Geometry check sheet. Reference: the model listing, model coordinates, mm. A direction names the side the tool comes from. Coordinates: 2 decimals unless noted, no trailing zeros. Order: outer loops, then holes, each group sorted by start corner. A loop starts at its lowest first (then second) coordinate and runs counter-clockwise, first axis right, second up. Notation, with made-up numbers: (-0.75, 32.5) - (52.25, 32.5) arc R14 cw to (52.25, 59.5) - close; hole circle Ø2 at (-35, 73.5). An arc over 180 degrees is marked (long way). Return JSON: item names as keys, results as strings. Group by question number.
Item 1: Section check C-C on x = -11. Enter the section's corners in (y, z), then the cut area to 3 significant figures.
Item 2: Gauge pin test, flat ends, axial feed: pin 1 (3.5 mm diameter, centred on x = -4.95, y = -4.95, fed in from +Z); pin 2 (1 mm diameter, centred on y = 0, z = 13, fed in from +X); pin 3 (4 mm diameter, centred on y = 10, z = 15.5, fed in from -X); pin 4 (2.5 mm diameter, centred on x = -8, z = 15, fed in from -Y). Record the tip position at first contact, or that the pin passes through.
Item 3: Scan lines: probe 1 along Y at (x, z) = (-1.4, 16); probe 2 along Y at (x, z) = (-5, 2.25); probe 3 along Y at (x, z) = (-0.75, 13.75). Record each from-to range of solid material in increasing order.
Item 4: Section check D-D on x = -2. Enter the section's corners in (y, z).
Item 5: Section check B-B on z = 16. Enter the section's corners in (x, y), then the cut area to 4 significant figures.
Item 6: Tool access check on faces 1 (the cylindrical face through (-10, 0, 7)), 2 (the flat face through (-4, 9.96, 14.98)), 3 (the flat face through (-5, 0, 14)). Record the directions out of +Z, -Z, +X, -X, +Y, -Y that give a thin tool (end or side, any length) a straight path to the whole face; none if there is none.
Item 7: Section check A-A on y = 10.5. Enter the section's corners in (x, z), then the cut area to 4 significant figures.
Item 8: Draft check along Y on faces 4 (the flat face through (-8, -7.5, 16)), 5 (the flat face through (-5, 0, 3)), 6 (the flat face through (0, 10.2, 8.9)). Enter one of: pulls with the +Y half, pulls with the -Y half, needs draft (parallel to the pull), parting line crosses it, or undercut.
from build123d import *

# Parameters (mm, degrees)
SKETCH_1_W               = 25
SKETCH_1_H               = 25
EXTRUDE_1_DEPTH          = 10
SKETCH_2_R               = 10
CUT_EXTRUDE_1_DEPTH      = 7
SKETCH_3_R               = 4.5
CUT_EXTRUDE_2_DEPTH      = 20.013153342
SKETCH_4_R               = 2
CUT_EXTRUDE_4_DEPTH      = 20.013153342
PATTERN_CIRCULAR_1_COUNT = 4
SKETCH_5_W               = 25
SKETCH_5_H               = 25
EXTRUDE_2_DEPTH          = 8
SKETCH_6_W               = 10
SKETCH_6_H               = 10
CUT_EXTRUDE_5_DEPTH      = 8
SKETCH_8_W               = 17.447834749
SKETCH_8_H               = 20.945056097
CUT_EXTRUDE_8_DEPTH      = 34.24530042
CUT_EXTRUDE_START        = -4
SKETCH_12_W              = 5
SKETCH_12_H              = 5
CUT_EXTRUDE_9_DEPTH      = 22.228951623
SKETCH_13_R              = 1
CUT_EXTRUDE_10_DEPTH     = 24.505318547


with BuildPart() as part:
    # 草图1 → 凸台-拉伸1 (new body)
    with BuildSketch(Plane.XY):
        Rectangle(SKETCH_1_W, SKETCH_1_H)
    extrude(amount=EXTRUDE_1_DEPTH)

    # 草图2 → 切除-拉伸1 (cut)
    with BuildSketch(Plane.XY.offset(10)):
        Circle(SKETCH_2_R)
    extrude(amount=-CUT_EXTRUDE_1_DEPTH, mode=Mode.SUBTRACT)

    # 草图3 → 切除-拉伸2 (cut, through all)
    with BuildSketch(Plane.XY.offset(3)):
        Circle(SKETCH_3_R)
    extrude(amount=-CUT_EXTRUDE_2_DEPTH, mode=Mode.SUBTRACT)

    # 草图4 → 切除-拉伸4 (cut, through all)
    with BuildSketch(Plane.XY.offset(3)):
        with Locations((-4.949747468, 4.949747468)):
            Circle(SKETCH_4_R)
    cut_extrude_4 = extrude(amount=-CUT_EXTRUDE_4_DEPTH, mode=Mode.SUBTRACT)

    # 阵列(圆周)1: 切除-拉伸4 ×4 about axis
    pattern_circular_1_axis = Axis((0, 0, 0), (0, 0, 1))
    for i in range(1, PATTERN_CIRCULAR_1_COUNT):
        add(cut_extrude_4.rotate(pattern_circular_1_axis, i * 360 / PATTERN_CIRCULAR_1_COUNT), mode=Mode.SUBTRACT)

    # 草图5 → 凸台-拉伸2 (add)
    with BuildSketch(Plane.XY.offset(10)):
        Rectangle(SKETCH_5_W, SKETCH_5_H)
    extrude(amount=EXTRUDE_2_DEPTH)

    # 草图6 → 切除-拉伸5 (cut)
    with BuildSketch(Plane.XY.offset(18)):
        Rectangle(SKETCH_6_W, SKETCH_6_H)
    extrude(amount=-CUT_EXTRUDE_5_DEPTH, mode=Mode.SUBTRACT)

    # 草图8 → 切除-拉伸8 (cut, through all)
    with BuildSketch(Plane.XZ.offset(12.5)):
        with Locations((8.723917375, 10.472528049)):
            Rectangle(SKETCH_8_W, SKETCH_8_H)
    extrude(amount=-CUT_EXTRUDE_8_DEPTH, mode=Mode.SUBTRACT)

    # 草图12 → 切除-拉伸9 (cut, through all)
    with BuildSketch(Plane(origin=(0, 0, 0), x_dir=(0, 0, -1), z_dir=(1, 0, 0)).offset(CUT_EXTRUDE_START)):
        with Locations((-15.5, -10)):
            Rectangle(SKETCH_12_W, SKETCH_12_H)
    cut_extrude_9 = extrude(amount=-CUT_EXTRUDE_9_DEPTH, mode=Mode.SUBTRACT)

    # 镜向1: 切除-拉伸9 across plane
    add(cut_extrude_9.mirror(Plane.ZX), mode=Mode.SUBTRACT)

    # 草图13 → 切除-拉伸10 (cut, through all)
    with BuildSketch(Plane.ZY.offset(4)):
        with Locations((16, -10.5)):
            Circle(SKETCH_13_R)
    cut_extrude_10 = extrude(amount=-CUT_EXTRUDE_10_DEPTH, mode=Mode.SUBTRACT)

    # 镜向2: 切除-拉伸10 across plane
    add(cut_extrude_10.mirror(Plane.ZX), mode=Mode.SUBTRACT)


solid = part.part
Computed:
{
 "1": {"outline": "(-12.5, 0) - (12.5, 0) - (12.5, 13) - (7.5, 13) - (7.5, 18) - (-7.5, 18) - (-7.5, 13) - (-12.5, 13) - close", "area": "400 mm²"},
 "2": {"pin 1": "stops at z = 18", "pin 2": "stops at x = -5", "pin 3": "stops at x = -4", "pin 4": "stops at y = -7.5"},
 "3": {"probe 1": "y = -12.5 to -11.5, -9.5 to -5, 5 to 9.5, 11.5 to 12.5", "probe 2": "y = -12.5 to -6.95, -2.95 to 2.95, 6.95 to 12.5", "probe 3": "y = -12.5 to -5, 5 to 12.5"},
 "4": {"outline": "(-12.5, 0) - (-4.03, 0) - (-4.03, 3) - (-9.8, 3) - (-9.8, 10) - (-5, 10) - (-5, 18) - (-12.5, 18) - close; (4.03, 0) - (12.5, 0) - (12.5, 18) - (5, 18) - (5, 10) - (9.8, 10) - (9.8, 3) - (4.03, 3) - close; hole circle Ø2 at (-10.5, 16); hole circle Ø2 at (10.5, 16)"},
 "5": {"outline": "(-12.5, -7.5) - (-4, -7.5) - (-4, -9.5) - (0, -9.5) - (0, -5) - (-5, -5) - (-5, 5) - (0, 5) - (0, 9.5) - (-4, 9.5) - (-4, 7.5) - (-12.5, 7.5) - close; (-4, -12.5) - (0, -12.5) - (0, -11.5) - (-4, -11.5) - close; (-4, 11.5) - (0, 11.5) - (0, 12.5) - (-4, 12.5) - close", "area": "161.5 mm²"},
 "6": {"face 1": "+X", "face 2": "+Z, -X, +Y", "face 3": "+Z, +X"},
 "7": {"outline": "(-12.5, 0) - (0, 0) - (0, 15) - (-4, 15) - (-4, 13) - (-12.5, 13) - close; (-4, 17) - (0, 17) - (0, 18) - (-4, 18) - close", "area": "174.5 mm²"},
 "8": {"face 4": "pulls with the -Y half", "face 5": "undercut", "face 6": "needs draft"}
}
